Check sheet for the modelled part. Datum: model origin and axes. Units: mm. Face numbers are marked on the shaded views. Round coordinates to 2 decimals unless told otherwise and drop trailing zeros. Order: outer loops, then holes, each group sorted by start corner. A loop starts at its lowest first (then second) coordinate and runs counter-clockwise, first axis right, second up. Notation, with made-up numbers: (-8.75, 79) -> (4.25, 79) arc R17 ccw to (4.25, 102) -> close; hole circle Ø5 at (10, -24). An arc over 180 degrees is marked (long way). Answer in a Markdown table with one row per item.
```python
from build123d import *

# Parameters (mm, degrees)
SKETCH_W     = 25
SKETCH_H     = 8
SKETCH_R     = 1.7
PAD_DEPTH    = 7
SKETCH002_R  = 4
POCKET_DEPTH = 8.001


with BuildPart() as part:
    # Sketch → Pad (new body)
    with BuildSketch(Plane.XY):
        with Locations((9.5, 0)):
            Rectangle(SKETCH_W, SKETCH_H)
        Circle(SKETCH_R, mode=Mode.SUBTRACT)
        with Locations((19, 0)):
            Circle(SKETCH_R, mode=Mode.SUBTRACT)
    extrude(amount=PAD_DEPTH)

    # Sketch002 → Pocket (cut, through all)
    with BuildSketch(Plane.XZ.offset(4)):
        with Locations((10, -1)):
            Circle(SKETCH002_R)
    extrude(amount=-POCKET_DEPTH, mode=Mode.SUBTRACT)


solid = part.part
```
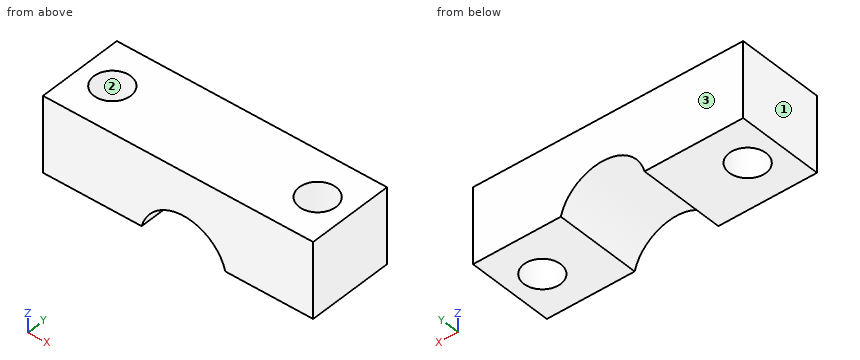
(1) Section check D-D on z = 1.5. Record the boundary of the cut face in (x, y), plus the area to 3 significant figures.
Solutions:
| item | result |
|---|---|
| outline | (-3, -4) -> (6.88, -4) -> (6.88, 4) -> (-3, 4) -> close; (13.12, -4) -> (22, -4) -> (22, 4) -> (13.12, 4) -> close; hole circle Ø3.4 at (0, 0); hole circle Ø3.4 at (19, 0) |
| area | 132 mm^2 |
(2) Section check C-C on z = 5.5. Record the boundary of the cut face in (x, y).
Solutions:
| item | result |
|---|---|
| outline | (-3, -4) -> (22, -4) -> (22, 4) -> (-3, 4) -> close; hole circle Ø3.4 at (0, 0); hole circle Ø3.4 at (19, 0) |
(3) Scan lines: probe 1 along Y at (x, z) = (19, 5.75); probe 2 along X at (y, z) = (0.25, 1); probe 3 along X at (y, z) = (-1, 6.5). Record each from-to range of solid material in increasing order. Write a range as from..to.
Solutions:
| item | result |
|---|---|
| probe 1 | -4..-1.7, 1.7..4 |
| probe 2 | -3..-1.68, 1.68..6.54, 13.46..17.32, 20.68..22 |
| probe 3 | -3..-1.37, 1.37..17.63, 20.37..22 |
(4) Section check B-B on y = 0. Record the boundary of the cut face in (x, z), plus the area to 3 significant figures.
Solutions:
| item | result |
|---|---|
| outline | (-3, 0) -> (-1.7, 0) -> (-1.7, 7) -> (-3, 7) -> close; (1.7, 0) -> (6.13, 0) arc R4 cw to (13.87, 0) -> (17.3, 0) -> (17.3, 7) -> (1.7, 7) -> close; (20.7, 0) -> (22, 0) -> (22, 7) -> (20.7, 7) -> close |
| area | 110 mm^2 |
(5) Draft check along Y on the marked faces 1, 2 and 3. Enter one of: pulls with the +Y half, pulls with the -Y half, needs draft (parallel to the pull), parting line crosses it, or undercut.
Solutions:
| item | result |
|---|---|
| face 1 | needs draft |
| face 2 | undercut |
| face 3 | pulls with the +Y half |
(6) Section check A-A on x = 0. Record the boundary of the cut face in (y, z).
Solutions:
| item | result |
|---|---|
| outline | (-4, 0) -> (-1.7, 0) -> (-1.7, 7) -> (-4, 7) -> close; (1.7, 0) -> (4, 0) -> (4, 7) -> (1.7, 7) -> close |
